Could you check a few things on this model? Use its own coordinates, in mm. Face numbers are marked on the shaded views. A direction names the side the tool comes from. Round coordinates to 2 decimals unless told otherwise and drop trailing zeros. Write each loop counter-clockwise with the first axis right and the second up, starting at its lowest first coordinate (ties: lowest second). Pieces come first, ordered by that corner, then holes. Notation, with made-up numbers: (-14.75, 21) -> (2.25, 21) arc R22 ccw to (2.25, 56) -> close; hole circle Ø11 at (-5.5, -14). An arc over 180 degrees is marked (long way). Answer as CSV lines item,"result". Start each with the question number.
Q1. Will these pins go through, and if not, where does the flat tip stop? pin 1 Ø1 at (x, y) = (12, 8) entering from +Z; pin 2 Ø5.5 at (x, y) = (23, 14) entering from +Z; pin 3 Ø1.8 at (x, y) = (35, 55.5) entering from +Z; pin 4 Ø0.9 at (x, y) = (22.5, 0.5) entering from +Z.
Q2. Imagine slicing it at B-B on x = 35. Please give me the cut outline in (y, z), and give its area (3 significant figures).
Q3. Imagine slicing it at D-D on y = 4.5. Please give me the cut outline in (x, z), and give its area (3 significant figures).
Q4. For the marked faces 4, 5 and 6, which set-ups out of +Z, -Z, +X, -X, +Y, -Y let a thin tool reach every point of the face, with its end or its side?
Q5. If I drill on line 1 (Y direction, x = 5, z = 4.5); line 2 (Y direction, x = 10, z = 7.5); line 3 (X direction, y = 25, z = 7), over which ranges is the centre line in solid material (lowest first)? Write a range as [from, to].
Q6. Imagine slicing it at C-C on x = 10. Please give me the cut outline in (y, z), and give its area (3 significant figures).
Q7. Imagine slicing it at A-A on y = 37. Please give me the cut outline in (x, z), and give its area (3 significant figures).
Q8. If we mould it in two halves opening along X, with no side actions, what happens to the marked faces 1, 2 and 3? For each: pulls with the +X half, pulls with the -X half, needs draft (parallel to the pull), parting line crosses it, or undercut.
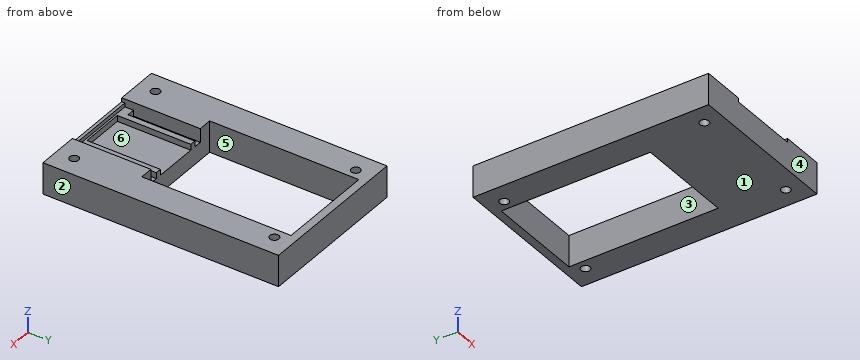
from build123d import *

# Parameters (mm, degrees)
SKETCH1_W           = 60
SKETCH1_H           = 40
BOSS_EXTRUDE1_DEPTH = 8
SKETCH3_R           = 1.15
CUT_EXTRUDE2_DEPTH  = 73.553428589
SKETCH7_W           = 25
SKETCH7_H           = 38
CUT_EXTRUDE6_DEPTH  = 73.553428589
SKETCH8_W           = 18.2
SKETCH8_H           = 45
CUT_EXTRUDE7_DEPTH  = 2
SKETCH9_W           = 2
SKETCH9_H           = 17
CUT_EXTRUDE8_DEPTH  = 1.5
SKETCH10_W          = 18.2
SKETCH10_H          = 0.8
BOSS_EXTRUDE2_DEPTH = 1
SKETCH11_W          = 11.2
SKETCH11_H          = 18.7
CUT_EXTRUDE9_DEPTH  = 1.5


with BuildPart() as part:
    # Sketch1 → Boss-Extrude1 (new body)
    with BuildSketch(Plane(origin=(0, 0, 0), x_dir=(0, 1, 0), z_dir=(0, 0, 1))):
        with Locations((30, -20)):
            Rectangle(SKETCH1_W, SKETCH1_H)
    extrude(amount=BOSS_EXTRUDE1_DEPTH)

    # Sketch3 → Cut-Extrude2 (cut, through all)
    with BuildSketch(Plane.XY.offset(8)):
        with Locations((5, 4.5)):
            Circle(SKETCH3_R)
        with Locations((35, 4.5)):
            Circle(SKETCH3_R)
        with Locations((5, 55.5)):
            Circle(SKETCH3_R)
        with Locations((35, 55.5)):
            Circle(SKETCH3_R)
    extrude(amount=-CUT_EXTRUDE2_DEPTH, mode=Mode.SUBTRACT)

    # Sketch7 → Cut-Extrude6 (cut, through all)
    with BuildSketch(Plane.XY.offset(8)):
        with Locations((20, 39)):
            Rectangle(SKETCH7_W, SKETCH7_H)
    extrude(amount=-CUT_EXTRUDE6_DEPTH, mode=Mode.SUBTRACT)

    # Sketch8 → Cut-Extrude7 (cut)
    with BuildSketch(Plane.XY.offset(8)):
        with Locations((20.062509857, 22.5)):
            Rectangle(SKETCH8_W, SKETCH8_H)
    extrude(amount=-CUT_EXTRUDE7_DEPTH, mode=Mode.SUBTRACT)

    # Sketch9 → Cut-Extrude8 (cut)
    with BuildSketch(Plane.XY.offset(6)):
        with Locations((11.962509857, 11.5)):
            Rectangle(SKETCH9_W, SKETCH9_H)
        with Locations((28.162509857, 11.5)):
            Rectangle(SKETCH9_W, SKETCH9_H)
    extrude(amount=-CUT_EXTRUDE8_DEPTH, mode=Mode.SUBTRACT)

    # Sketch10 → Boss-Extrude2 (add)
    with BuildSketch(Plane.XY.offset(6)):
        with Locations((20.062509857, 0.4)):
            Rectangle(SKETCH10_W, SKETCH10_H)
    extrude(amount=BOSS_EXTRUDE2_DEPTH)

    # Sketch11 → Cut-Extrude9 (cut)
    with BuildSketch(Plane.XY.offset(6)):
        with Locations((20.062509857, 10.65)):
            Rectangle(SKETCH11_W, SKETCH11_H)
    extrude(amount=-CUT_EXTRUDE9_DEPTH, mode=Mode.SUBTRACT)


solid = part.part
Checks:
1,pin 1,"z = 4.5"
1,pin 2,"z = 6"
1,pin 3,"through"
1,pin 4,"z = 7"
2,outline,"(0, 0) -> (3.35, 0) -> (3.35, 8) -> (0, 8) -> close; (5.65, 0) -> (54.35, 0) -> (54.35, 8) -> (5.65, 8) -> close; (56.65, 0) -> (60, 0) -> (60, 8) -> (56.65, 8) -> close"
2,area,"443 mm^2"
3,outline,"(0, 0) -> (3.85, 0) -> (3.85, 8) -> (0, 8) -> close; (6.15, 0) -> (33.85, 0) -> (33.85, 8) -> (29.16, 8) -> (29.16, 4.5) -> (27.16, 4.5) -> (27.16, 6) -> (25.66, 6) -> (25.66, 4.5) -> (14.46, 4.5) -> (14.46, 6) -> (12.96, 6) -> (12.96, 4.5) -> (10.96, 4.5) -> (10.96, 8) -> (6.15, 8) -> close; (36.15, 0) -> (40, 0) -> (40, 8) -> (36.15, 8) -> close"
3,area,"224 mm^2"
4,face 4,"+Z, -Z, +X, -X, -Y"
4,face 5,"+Z, -Z"
4,face 6,"+Z"
5,line 1,"[0, 3.35], [5.65, 54.35], [56.65, 60]"
5,line 2,"[0, 20], [58, 60]"
5,line 3,"[0, 7.5], [32.5, 40]"
6,outline,"(0, 0) -> (20, 0) -> (20, 8) -> (0, 8) -> close; (58, 0) -> (60, 0) -> (60, 8) -> (58, 8) -> close"
6,area,"176 mm^2"
7,outline,"(0, 0) -> (7.5, 0) -> (7.5, 8) -> (0, 8) -> close; (32.5, 0) -> (40, 0) -> (40, 8) -> (32.5, 8) -> close"
7,area,"120 mm^2"
8,face 1,"needs draft"
8,face 2,"pulls with the +X half"
8,face 3,"undercut"
